Source: three-view drawing plus pictorial views. Frame: mm from the lowest corner of the part. A direction names the side the tool comes from. Give positions to 0.01 mm unless a question says otherwise; leave off trailing zeros. Loops run counter-clockwise (first coordinate to the right, second up) from the corner with the lowest first, then second, coordinate; pieces in that order, holes last. Notation, with made-up numbers: (77.5, 20) -> (95.5, 20) arc R22 ccw to (95.5, 59) -> close; hole circle Ø1 at (-18, -14). An arc over 180 degrees is marked (long way). Answer as a JSON object with one key per item and string values. Group by question number.
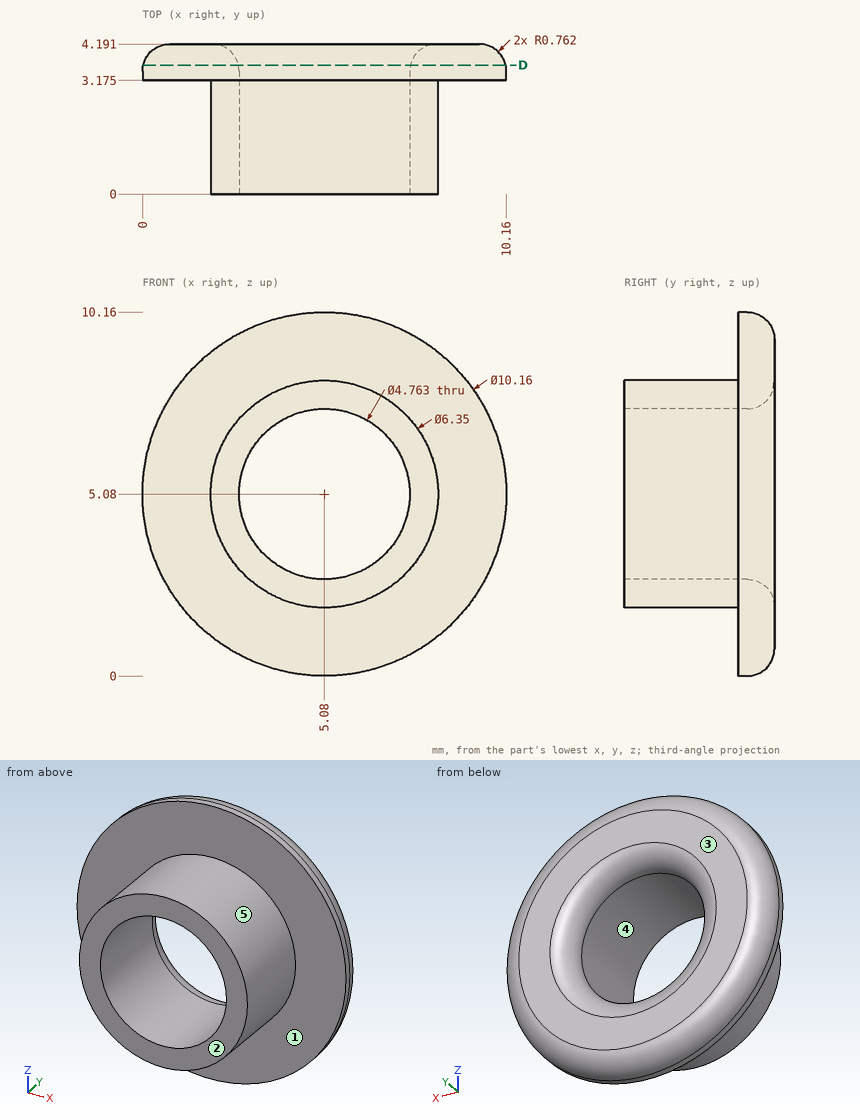
Q1. Pull-direction query (X, two-part tool) for the marked faces 3, 4 and 5; classes: +X half, -X half, draft (parallel to the pull), parting line (faces both ways), or undercut.
Q2. Pin query (flat end, axial travel): pin 1 Ø1 at (x, z) = (3.5, 3) entering from -Y; pin 2 Ø1 at (x, y) = (3, 0.5) entering from +Z (1 decimal). Return the tip coordinate at first contact, or that it passes through.
Q3. Ray query, probe 1 along Z at (x, y) = (5.08, 1.9) (1 decimal); probe 2 along Y at (x, z) = (2, 8) (1 decimal). Return the intervals inside material, ascending.
Q4. Set-up query: the marked faces 1 and 2. Return all of +Z, -Z, +X, -X, +Y, -Y with unobstructed straight access to the full face (end or side cutting, diameter ignored); none if empty.
Q5. Section D-D on y = 3.6. Return the cut outline in (x, z).
Numbers:
{
 "1": {"face 3": "draft", "face 4": "undercut", "face 5": "parting line"},
 "2": {"pin 1": "stops at y = 0", "pin 2": "stops at z = 7.8"},
 "3": {"probe 1": "z = 1.9 to 2.7, 7.5 to 8.3", "probe 2": "y = 3.2 to 4.2"},
 "4": {"face 1": "-Y", "face 2": "+Z, -Z, +X, -X, -Y"},
 "5": {"outline": "circle Ø10.12 at (5.08, 5.08); hole circle Ø4.8 at (5.08, 5.08)"}
}
